Could you check a few things on this model? Use its own coordinates, in mm. Give positions to 0.01 mm unless a question says otherwise; leave off trailing zeros. Write each loop counter-clockwise with the first axis right and the second up, starting at its lowest first coordinate (ties: lowest second). Pieces come first, ordered by that corner, then holes. Notation, with made-up numbers: (-36, 69.25) - (0, 69.25) arc R34 cw to (0, 108.25) - close; hole circle Ø7 at (-36.75, 67.25). An arc over 180 degrees is marked (long way). Answer as CSV lines item,"result". Start each with the question number.
Q1. Imagine slicing it at A-A on y = 17.5. List the corners of the cut face in (x, z) for me, and give its area (3 significant figures).
Q2. If I drill on line 1 along X through (y, z) = (-17.5, 1.35); line 2 along Y through (x, z) = (7, 1.15); line 3 along X through (y, z) = (-18.5, 1.75), over which ranges is the centre line in solid material (lowest first)?
Q3. Will these pins go through, and if not, where does the flat tip stop? pin 1 Ø1 at (y, z) = (9, 1.5) entering from +X; pin 2 Ø8 at (x, y) = (7, -18.5) entering from -Z.
Q4. Imagine slicing it at D-D on x = 5. List the corners of the cut face in (y, z) for me.
Q5. Imagine slicing it at C-C on z = 1.4. State how many separate pieces and enclosed holes the cut face has, and give its area (3 significant figures).
```python
from build123d import *

# Parameters (mm, degrees)
F1_DEPTH = 2


with BuildPart() as f1:
    # F0 (on Top) → F1 (new body)
    with BuildSketch(Plane.XY):
        Polygon((1.220858, 23.295364), (0, 20.827976), (-1.220858, 23.295364), (-2.177116, 20.713879), (-3.649199, 23.040135), (-4.33038, 20.372835), (-6.037558, 22.532474), (-6.436199, 19.808583), (-8.359769, 21.777942), (-8.471501, 19.027303), (-10.590388, 20.784806), (-10.413988, 18.037557), (-12.704976, 19.563948), (-12.242377, 16.850187), (-14.680367, 18.128743), (-13.936636, 15.478203), (-16.494916, 16.494916), (-15.478203, 13.936636), (-18.128743, 14.680367), (-16.850187, 12.242377), (-19.563948, 12.704976), (-18.037557, 10.413988), (-20.784806, 10.590388), (-19.027303, 8.471501), (-21.777942, 8.359769), (-19.808583, 6.436199), (-22.532474, 6.037558), (-20.372835, 4.33038), (-23.040135, 3.649199), (-20.713879, 2.177116), (-23.295364, 1.220858), (-20.827976, 0), (-23.295364, -1.220858), (-20.713879, -2.177116), (-23.040135, -3.649199), (-20.372835, -4.33038), (-22.532474, -6.037558), (-19.808583, -6.436199), (-21.777942, -8.359769), (-19.027303, -8.471501), (-20.784806, -10.590388), (-18.037557, -10.413988), (-19.563948, -12.704976), (-16.850187, -12.242377), (-18.128743, -14.680367), (-15.478203, -13.936636), (-16.494916, -16.494916), (-13.936636, -15.478203), (-14.680367, -18.128743), (-12.242377, -16.850187), (-12.704976, -19.563948), (-10.413988, -18.037557), (-10.590388, -20.784806), (-8.471501, -19.027303), (-8.359769, -21.777942), (-6.436199, -19.808583), (-6.037558, -22.532474), (-4.33038, -20.372835), (-3.649199, -23.040135), (-2.177116, -20.713879), (-1.220858, -23.295364), (0, -20.827976), (1.220858, -23.295364), (2.177116, -20.713879), (3.649199, -23.040135), (4.33038, -20.372835), (6.037558, -22.532474), (6.436199, -19.808583), (8.359769, -21.777942), (8.471501, -19.027303), (10.590388, -20.784806), (10.413988, -18.037557), (12.704976, -19.563948), (12.242377, -16.850187), (14.680367, -18.128743), (13.936636, -15.478203), (16.494916, -16.494916), (15.478203, -13.936636), (18.128743, -14.680367), (16.850187, -12.242377), (19.563948, -12.704976), (18.037557, -10.413988), (20.784806, -10.590388), (19.027303, -8.471501), (21.777942, -8.359769), (19.808583, -6.436199), (22.532474, -6.037558), (20.372835, -4.33038), (23.040135, -3.649199), (20.713879, -2.177116), (23.295364, -1.220858), (20.827976, 0), (23.295364, 1.220858), (20.713879, 2.177116), (23.040135, 3.649199), (20.372835, 4.33038), (22.532474, 6.037558), (19.808583, 6.436199), (21.777942, 8.359769), (19.027303, 8.471501), (20.784806, 10.590388), (18.037557, 10.413988), (19.563948, 12.704976), (16.850187, 12.242377), (18.128743, 14.680367), (15.478203, 13.936636), (16.494916, 16.494916), (13.936636, 15.478203), (14.680367, 18.128743), (12.242377, 16.850187), (12.704976, 19.563948), (10.413988, 18.037557), (10.590388, 20.784806), (8.471501, 19.027303), (8.359769, 21.777942), (6.436199, 19.808583), (6.037558, 22.532474), (4.33038, 20.372835), (3.649199, 23.040135), (2.177116, 20.713879), align=None)
        with BuildLine():
            Line((-2.414022, -0.65), (2.414022, -0.65))
            ThreePointArc((2.414022, -0.65), (0, -2.5), (-2.414022, -0.65))
        make_face(mode=Mode.SUBTRACT)
        with BuildLine():
            ThreePointArc((-2.414022, 0.65), (0, 2.5), (2.414022, 0.65))
            Line((2.414022, 0.65), (-2.414022, 0.65))
        make_face(mode=Mode.SUBTRACT)
    extrude(amount=F1_DEPTH)


solid = f1.part
```
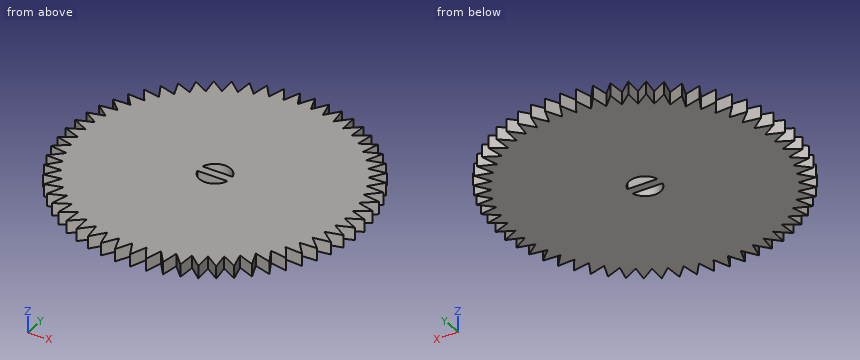
Conclusion:
1,outline,"(-14.5, 0) - (-13.48, 0) - (-13.48, 2) - (-14.5, 2) - close; (-12.35, 0) - (12.35, 0) - (12.35, 2) - (-12.35, 2) - close; (13.48, 0) - (14.5, 0) - (14.5, 2) - (13.48, 2) - close"
1,area,"53.5 mm^2"
2,line 1,"-14.5 to -13.48, -12.35 to 12.35, 13.48 to 14.5"
2,line 2,"-20.39 to 20.39"
2,line 3,"-12.52 to -11.11, -10.44 to 10.44, 11.11 to 12.52"
3,pin 1,"x = 19.88"
3,pin 2,"z = 0"
4,outline,"(-21.22, 0) - (21.22, 0) - (21.22, 2) - (-21.22, 2) - close"
5,separate pieces,"1"
5,enclosed holes,"2"
5,area,"1,510 mm^2"
